Read the model definition and answer for the solid it produces. Units are mm, in the model's axes. A direction names the side the tool comes from. Coordinates: 2 decimals unless noted, no trailing zeros. Loops run counter-clockwise (first coordinate to the right, second up) from the corner with the lowest first, then second, coordinate; pieces in that order, holes last. Notation, with made-up numbers: (-36, 43) -> (-10, 43) arc R19 cw to (-10, 51) -> close; hole circle Ø8 at (31.25, 14.5). An arc over 180 degrees is marked (long way). Answer as a JSON object with one key per item and string values. Group by question number.
1) Section B-B, the plane x = 27 is taken. Give the vertices of the cut face in (y, z), plus the area to 3 significant figures.
2) Section C-C, the plane y = -11.5 is taken. Give the vertices of the cut face in (x, z).
3) Consider probe 1 along Y at (x, z) = (34, 19); probe 2 along Z at (x, y) = (37.5, -12.25); probe 3 along X at (y, z) = (13, 13). Determine where each line is inside the solid, lowest interval first. Write a range as [from, to].
4) Section D-D, the plane z = 17.5 is taken. Give the vertices of the cut face in (x, y).
5) Section A-A, the plane z = 7 is taken. Give the vertices of the cut face in (x, y), plus the area to 3 significant figures.
6) Which of the six approach directions +Z, -Z, +X, -X, +Y, -Y give full straight-line access (tool end or side, diameter ignored) to faces 1 (the face through (40, 14.2, 15)), 2 (the face through (32.621, -12, 15)), 3 (the face through (51.821, -12, 11))?
7) Flat-ended cylindrical pins translate along their axes: P1, Ø2, axis at x = 50, z = 12.5, coming from the +Y side; P2, Ø2.5, axis at x = 27, y = -11.5, coming from the -Z side; P3, Ø8, axis at x = 51.5, y = -2, coming from the +Z side; P4, Ø2, axis at y = 11, z = 10.5, coming from the +X side. Find the tip coordinate at first contact, or state that the pin passes through.
8) Determine the mould class of faces 4 (the face through (42.621, 12, 18)), 5 (the face through (42, 0, 8)), 6 (the face through (32.621, 12, 15)) for opening direction X: released by +X, released by -X, zero draft, split by the parting line, or undercut.
from build123d import *

# Parameters (mm, degrees)
REMOVABLE_ADAPTER_BASE_START           = 4
REMOVABLE_ADAPTER_BASE_PROFILE_W       = 39
REMOVABLE_ADAPTER_BASE_PROFILE_H       = 30
REMOVABLE_ADAPTER_BASE_DEPTH           = 4
LEFT_PIN0_SUPPORT_START                = 10.2
LEFT_PIN0_SUPPORT_PROFILE_W            = 10
LEFT_PIN0_SUPPORT_PROFILE_H            = 13
LEFT_PIN0_SUPPORT_DEPTH                = 4
LEFT_PIN0_ROUNDED_LUG_START            = 10.2
LEFT_PIN0_ROUNDED_LUG_PROFILE_R        = 5
LEFT_PIN0_ROUNDED_LUG_DEPTH            = 4
LEFT_PIN1_SUPPORT_START                = 10.2
LEFT_PIN1_SUPPORT_PROFILE_W            = 10
LEFT_PIN1_SUPPORT_PROFILE_H            = 5
LEFT_PIN1_SUPPORT_DEPTH                = 4
LEFT_PIN1_ROUNDED_LUG_START            = 10.2
LEFT_PIN1_ROUNDED_LUG_PROFILE_R        = 5
LEFT_PIN1_ROUNDED_LUG_DEPTH            = 4
RIGHT_PIN0_SUPPORT_START               = -14.2
RIGHT_PIN0_SUPPORT_PROFILE_W           = 10
RIGHT_PIN0_SUPPORT_PROFILE_H           = 13
RIGHT_PIN0_SUPPORT_DEPTH               = 4
RIGHT_PIN0_ROUNDED_LUG_START           = -14.2
RIGHT_PIN0_ROUNDED_LUG_PROFILE_R       = 5
RIGHT_PIN0_ROUNDED_LUG_DEPTH           = 4
RIGHT_PIN1_SUPPORT_START               = -14.2
RIGHT_PIN1_SUPPORT_PROFILE_W           = 10
RIGHT_PIN1_SUPPORT_PROFILE_H           = 5
RIGHT_PIN1_SUPPORT_DEPTH               = 4
RIGHT_PIN1_ROUNDED_LUG_START           = -14.2
RIGHT_PIN1_ROUNDED_LUG_PROFILE_R       = 5
RIGHT_PIN1_ROUNDED_LUG_DEPTH           = 4
BOTH_M4_GRIPPER_PIN_AXES_START         = -20
BOTH_M4_GRIPPER_PIN_AXES_PROFILE_R     = 2.15
BOTH_M4_GRIPPER_PIN_AXES_DEPTH         = 89.883960397
FOUR_M3_REMOVABLE_DECK_BOLTS_START     = -50
FOUR_M3_REMOVABLE_DECK_BOLTS_PROFILE_R = 1.7
FOUR_M3_REMOVABLE_DECK_BOLTS_DEPTH     = 119.883960397


with BuildPart() as part:
    # Removable_adapter_base_profile → Removable_adapter_base (new body)
    with BuildSketch(Plane.XY.offset(REMOVABLE_ADAPTER_BASE_START)):
        with Locations((42.5, 0)):
            Rectangle(REMOVABLE_ADAPTER_BASE_PROFILE_W, REMOVABLE_ADAPTER_BASE_PROFILE_H)
    extrude(amount=REMOVABLE_ADAPTER_BASE_DEPTH)

    # Left_pin0_support_profile → Left_pin0_support (add)
    with BuildSketch(Plane(origin=(0, 0, 0), x_dir=(1, 0, 0), z_dir=(0, 1, 0)).offset(LEFT_PIN0_SUPPORT_START)):
        with Locations((37.620525892, -14.5)):
            Rectangle(LEFT_PIN0_SUPPORT_PROFILE_W, LEFT_PIN0_SUPPORT_PROFILE_H)
    extrude(amount=LEFT_PIN0_SUPPORT_DEPTH)

    # Left_pin0_rounded_lug_profile → Left_pin0_rounded_lug (add)
    with BuildSketch(Plane(origin=(0, 0, 0), x_dir=(1, 0, 0), z_dir=(0, 1, 0)).offset(LEFT_PIN0_ROUNDED_LUG_START)):
        with Locations((37.620525892, -21)):
            Circle(LEFT_PIN0_ROUNDED_LUG_PROFILE_R)
    extrude(amount=LEFT_PIN0_ROUNDED_LUG_DEPTH)

    # Left_pin1_support_profile → Left_pin1_support (add)
    with BuildSketch(Plane(origin=(0, 0, 0), x_dir=(1, 0, 0), z_dir=(0, 1, 0)).offset(LEFT_PIN1_SUPPORT_START)):
        with Locations((46.820525892, -10.5)):
            Rectangle(LEFT_PIN1_SUPPORT_PROFILE_W, LEFT_PIN1_SUPPORT_PROFILE_H)
    extrude(amount=LEFT_PIN1_SUPPORT_DEPTH)

    # Left_pin1_rounded_lug_profile → Left_pin1_rounded_lug (add)
    with BuildSketch(Plane(origin=(0, 0, 0), x_dir=(1, 0, 0), z_dir=(0, 1, 0)).offset(LEFT_PIN1_ROUNDED_LUG_START)):
        with Locations((46.820525892, -13)):
            Circle(LEFT_PIN1_ROUNDED_LUG_PROFILE_R)
    extrude(amount=LEFT_PIN1_ROUNDED_LUG_DEPTH)

    # Right_pin0_support_profile → Right_pin0_support (add)
    with BuildSketch(Plane(origin=(0, 0, 0), x_dir=(1, 0, 0), z_dir=(0, 1, 0)).offset(RIGHT_PIN0_SUPPORT_START)):
        with Locations((37.620525892, -14.5)):
            Rectangle(RIGHT_PIN0_SUPPORT_PROFILE_W, RIGHT_PIN0_SUPPORT_PROFILE_H)
    extrude(amount=RIGHT_PIN0_SUPPORT_DEPTH)

    # Right_pin0_rounded_lug_profile → Right_pin0_rounded_lug (add)
    with BuildSketch(Plane(origin=(0, 0, 0), x_dir=(1, 0, 0), z_dir=(0, 1, 0)).offset(RIGHT_PIN0_ROUNDED_LUG_START)):
        with Locations((37.620525892, -21)):
            Circle(RIGHT_PIN0_ROUNDED_LUG_PROFILE_R)
    extrude(amount=RIGHT_PIN0_ROUNDED_LUG_DEPTH)

    # Right_pin1_support_profile → Right_pin1_support (add)
    with BuildSketch(Plane(origin=(0, 0, 0), x_dir=(1, 0, 0), z_dir=(0, 1, 0)).offset(RIGHT_PIN1_SUPPORT_START)):
        with Locations((46.820525892, -10.5)):
            Rectangle(RIGHT_PIN1_SUPPORT_PROFILE_W, RIGHT_PIN1_SUPPORT_PROFILE_H)
    extrude(amount=RIGHT_PIN1_SUPPORT_DEPTH)

    # Right_pin1_rounded_lug_profile → Right_pin1_rounded_lug (add)
    with BuildSketch(Plane(origin=(0, 0, 0), x_dir=(1, 0, 0), z_dir=(0, 1, 0)).offset(RIGHT_PIN1_ROUNDED_LUG_START)):
        with Locations((46.820525892, -13)):
            Circle(RIGHT_PIN1_ROUNDED_LUG_PROFILE_R)
    extrude(amount=RIGHT_PIN1_ROUNDED_LUG_DEPTH)

    # Both_M4_gripper_pin_axes_profile → Both_M4_gripper_pin_axes (cut, through all)
    with BuildSketch(Plane(origin=(0, 0, 0), x_dir=(1, 0, 0), z_dir=(0, 1, 0)).offset(BOTH_M4_GRIPPER_PIN_AXES_START)):
        with Locations(Location((37.620525892, -21, 0), (0, 0, 90))):
            Circle(BOTH_M4_GRIPPER_PIN_AXES_PROFILE_R)
        with Locations(Location((46.820525892, -13, 0), (0, 0, 90))):
            Circle(BOTH_M4_GRIPPER_PIN_AXES_PROFILE_R)
    extrude(amount=BOTH_M4_GRIPPER_PIN_AXES_DEPTH, mode=Mode.SUBTRACT)

    # Four_M3_removable_deck_bolts_profile → Four_M3_removable_deck_bolts (cut, through all)
    with BuildSketch(Plane.XY.offset(FOUR_M3_REMOVABLE_DECK_BOLTS_START)):
        with Locations(Location((27, -11.5, 0), (0, 0, 180))):
            Circle(FOUR_M3_REMOVABLE_DECK_BOLTS_PROFILE_R)
        with Locations(Location((27, 11.5, 0), (0, 0, 180))):
            Circle(FOUR_M3_REMOVABLE_DECK_BOLTS_PROFILE_R)
        with Locations(Location((58, -11.5, 0), (0, 0, 180))):
            Circle(FOUR_M3_REMOVABLE_DECK_BOLTS_PROFILE_R)
        with Locations(Location((58, 11.5, 0), (0, 0, 180))):
            Circle(FOUR_M3_REMOVABLE_DECK_BOLTS_PROFILE_R)
    extrude(amount=FOUR_M3_REMOVABLE_DECK_BOLTS_DEPTH, mode=Mode.SUBTRACT)


solid = part.part
Determined:
{
 "1": {"outline": "(-15, 4) -> (-13.2, 4) -> (-13.2, 8) -> (-15, 8) -> close; (-9.8, 4) -> (9.8, 4) -> (9.8, 8) -> (-9.8, 8) -> close; (13.2, 4) -> (15, 4) -> (15, 8) -> (13.2, 8) -> close", "area": "92.8 mm²"},
 "2": {"outline": "(23, 4) -> (25.3, 4) -> (25.3, 8) -> (23, 8) -> close; (28.7, 4) -> (56.3, 4) -> (56.3, 8) -> (51.82, 8) -> (51.82, 13) arc R5 ccw to (42.62, 15.71) -> (42.62, 21) arc R5 ccw to (32.62, 21) -> (32.62, 8) -> (28.7, 8) -> close; (59.7, 4) -> (62, 4) -> (62, 8) -> (59.7, 8) -> close; hole circle Ø4.3 at (37.62, 21); hole circle Ø4.3 at (46.82, 13)"},
 "3": {"probe 1": "[-14.2, -10.2], [10.2, 14.2]", "probe 2": "[4, 18.85], [23.15, 26]", "probe 3": "[32.62, 44.67], [48.97, 51.82]"},
 "4": {"outline": "(32.62, -14.2) -> (42.62, -14.2) -> (42.62, -10.2) -> (32.62, -10.2) -> close; (32.62, 10.2) -> (42.62, 10.2) -> (42.62, 14.2) -> (32.62, 14.2) -> close; (44.64, -14.2) -> (49, -14.2) -> (49, -10.2) -> (44.64, -10.2) -> close; (44.64, 10.2) -> (49, 10.2) -> (49, 14.2) -> (44.64, 14.2) -> close"},
 "5": {"outline": "(23, -15) -> (62, -15) -> (62, 15) -> (23, 15) -> close; hole circle Ø3.4 at (27, -11.5); hole circle Ø3.4 at (27, 11.5); hole circle Ø3.4 at (58, -11.5); hole circle Ø3.4 at (58, 11.5)", "area": "1,130 mm²"},
 "6": {"face 1": "+Z, +X, -X, +Y", "face 2": "+Z, -X, +Y, -Y", "face 3": "+Z, +X, +Y, -Y"},
 "7": {"P1": "y = 14.2", "P2": "through", "P3": "z = 8", "P4": "x = 51.82"},
 "8": {"face 4": "undercut", "face 5": "zero draft", "face 6": "released by -X"}
}
